Autodesk Inventor part; units mm, degrees
ref_plane "YZ Plane" through (0, 0, 0) normal (1, 0, 0) x (0, 1, 0)
ref_plane "XZ Plane" through (0, 0, 0) normal (0, 1, 0) x (-1, 0, 0)
ref_plane "XY Plane" through (0, 0, 0) normal (0, 0, 1) x (1, 0, 0)
sketch "Sketch1" plane through (0, 0, 0) normal (0, 0, 1) x (1, 0, 0)
  line L0 (0, 0) -> (68.58, 0)
  line L1 (68.58, 0) -> (68.58, 107.95)
  line L2 (68.58, 107.95) -> (0, 107.95)
  line L3 (0, 107.95) -> (0, 0)
  dimension "d0" = 68.58
  dimension "d1" = 107.95
extrude "Extrusion1" add sketch "Sketch1" along normal blind 10
sketch "Sketch2" plane through (0, 0, 10) normal (0, 0, 1) x (1, 0, 0)
  circle A0 centre (34.29, 35.56) radius 30.48
  line L0 (0, 0) -> (68.58, 0)
  line L1 (68.58, 107.95) -> (0, 107.95)
  line L2 (25.1206, 107.95) -> (43.4594, 107.95)
  line L3 (43.4594, 107.95) -> (43.4594, 64.6281)
  line L4 (43.4594, 64.6281) -> (25.1206, 64.6281)
  line L5 (25.1206, 64.6281) -> (25.1206, 107.95)
  circle A1 centre (60.6865, 20.32) radius 5
  circle A2 centre (7.8935, 20.32) radius 5
  line L6 (7.8935, 20.32) -> (34.29, 66.04) construction
  line L7 (34.29, 66.04) -> (60.6865, 20.32) construction
  line L8 (60.6865, 20.32) -> (7.8935, 20.32) construction
  point P0 (34.29, 0)
  point P1 (34.29, 107.95)
  point P2 (57.8397, 16.2095)
  point P3 (62.8229, 24.8406)
  point P4 (10.7403, 16.2095)
  point P5 (5.7571, 24.8406)
  dimension "d4" = 18.3388
  dimension "d5" = 60.96
  dimension "d6" = 35.56
  dimension "d9" = 10
extrude "Extrusion2" cut sketch "Sketch2" against normal blind 7
sketch "Sketch4" plane through (0, 0, 3) normal (0, 0, 1) x (1, 0, 0)
  arc A0 (25.1206, 64.6281) -> (5.7571, 24.8406) centre (34.29, 35.56) ccw
  arc A1 (5.7571, 24.8406) -> (10.7403, 16.2095) centre (7.8935, 20.32) ccw
  arc A2 (10.7403, 16.2095) -> (57.8397, 16.2095) centre (34.29, 35.56) ccw
  arc A3 (57.8397, 16.2095) -> (62.8229, 24.8406) centre (60.6865, 20.32) ccw
  arc A4 (62.8229, 24.8406) -> (43.4594, 64.6281) centre (34.29, 35.56) ccw
  line L0 (43.4594, 107.95) -> (43.4594, 64.6281)
  line L1 (25.1206, 107.95) -> (43.4594, 107.95)
  line L2 (25.1206, 64.6281) -> (25.1206, 107.95)
  line L3 (25.1206, 64.6281) -> (25.1206, 107.95)
  line L4 (43.4594, 107.95) -> (43.4594, 64.6281)
  line L5 (25.1206, 107.95) -> (43.4594, 107.95)
  line L6 (43.4594, 107.95) -> (43.4594, 69.85)
  line L7 (43.4594, 69.85) -> (25.1206, 69.85)
  line L8 (25.1206, 69.85) -> (25.1206, 107.95)
  line L9 (25.1206, 107.95) -> (43.4594, 107.95)
  line L10 (28.1206, 107.95) -> (40.4594, 107.95)
  line L11 (40.4594, 107.95) -> (40.4594, 69.85)
  line L12 (40.4594, 69.85) -> (28.1206, 69.85)
  line L13 (28.1206, 69.85) -> (28.1206, 107.95)
  point P0 (0, 0)
  dimension "d17" = 3
  dimension "d18" = 3
  dimension "d19" = 38.1
extrude "Extrusion4" add sketch "Sketch4" along normal blind 3 contours L13 L1 L11 L7
sketch "Sketch3" plane through (0, 0, 3) normal (0, 0, 1) x (1, 0, 0)
  arc A0 (25.1206, 64.6281) -> (5.7571, 24.8406) centre (34.29, 35.56) ccw
  arc A1 (5.7571, 24.8406) -> (10.7403, 16.2095) centre (7.8935, 20.32) ccw
  arc A2 (10.7403, 16.2095) -> (57.8397, 16.2095) centre (34.29, 35.56) ccw
  arc A3 (57.8397, 16.2095) -> (62.8229, 24.8406) centre (60.6865, 20.32) ccw
  arc A4 (62.8229, 24.8406) -> (43.4594, 64.6281) centre (34.29, 35.56) ccw
  line L0 (43.4594, 107.95) -> (43.4594, 64.6281)
  line L1 (25.1206, 107.95) -> (28.1206, 107.95)
  line L2 (25.1206, 64.6281) -> (25.1206, 107.95)
  line L3 (25.1206, 64.6281) -> (25.1206, 107.95)
  line L4 (25.1206, 107.95) -> (43.4594, 107.95)
  line L5 (43.4594, 107.95) -> (43.4594, 106.95)
  line L6 (43.4594, 106.95) -> (25.1206, 106.95)
  line L7 (25.1206, 106.95) -> (25.1206, 107.95)
  line L8 (40.4594, 107.95) -> (40.4594, 69.85)
  line L9 (40.4594, 69.85) -> (28.1206, 69.85)
  line L10 (28.1206, 69.85) -> (28.1206, 107.95)
  line L11 (40.4594, 107.95) -> (43.4594, 107.95)
  point P0 (0, 0)
  point P1 (40.4594, 106.95)
  point P2 (28.1206, 106.95)
  dimension "d10" = 1
extrude "Extrusion3" add sketch "Sketch3" along normal blind 4.5 contours L2 L1 L10 L6 | L10 L4 L8 L6 | L8 L4 L0 L6
fillet "Fillet1" radius 5 4 edges at (0, 107.95, 5) (68.58, 107.95, 5) (68.58, 0, 5) (0, 0, 5)
chamfer "Chamfer1" distance 2 angle 45 8 edges at (34.29, 107.95, 0) (1.4645, 106.4855, 0) (0, 53.975, 0) (1.4645, 1.4645, 0) (34.29, 0, 0) (67.1155, 1.4645, 0) (68.58, 53.975, 0) (67.1155, 106.4855, 0)
sketch "Sketch6" plane through (0, 0, 10) normal (0, 0, 1) x (1, 0, 0)
  arc A0 (0, 5) -> (5, 0) centre (5, 5) ccw
  line L0 (5, 0) -> (63.58, 0)
  arc A1 (63.58, 0) -> (68.58, 5) centre (63.58, 5) ccw
  line L1 (68.58, 5) -> (68.58, 102.95)
  arc A2 (68.58, 102.95) -> (63.58, 107.95) centre (63.58, 102.95) ccw
  line L2 (63.58, 107.95) -> (43.4594, 107.95)
  line L3 (43.4594, 107.95) -> (43.4594, 64.6281)
  arc A3 (62.8229, 24.8406) -> (43.4594, 64.6281) centre (34.29, 35.56) ccw
  arc A4 (57.8397, 16.2095) -> (62.8229, 24.8406) centre (60.6865, 20.32) ccw
  arc A5 (10.7403, 16.2095) -> (57.8397, 16.2095) centre (34.29, 35.56) ccw
  arc A6 (5.7571, 24.8406) -> (10.7403, 16.2095) centre (7.8935, 20.32) ccw
  arc A7 (25.1206, 64.6281) -> (5.7571, 24.8406) centre (34.29, 35.56) ccw
  line L4 (25.1206, 64.6281) -> (25.1206, 107.95)
  line L5 (25.1206, 107.95) -> (5, 107.95)
  arc A8 (5, 107.95) -> (0, 102.95) centre (5, 102.95) ccw
  line L6 (0, 102.95) -> (0, 5)
  point P0 (0, 0)
hole "Hole2" at (5, 102.95, 10) at (5, 5, 10) at (63.58, 5, 10) at (63.58, 102.95, 10) direction (0, 0, -1) diameter 4 depth 6
sketch "Sketch7" plane through (25.1206, 107.95, 7.5) normal (0, 1, 0) x (1, 0, 0)
  line L0 (3.6694, -5.25) -> (14.6694, -5.25)
  line L1 (14.6694, -5.25) -> (14.6694, 2.75)
  line L2 (14.6694, 2.75) -> (3.6694, 2.75)
  line L3 (3.6694, 2.75) -> (3.6694, -5.25)
  line L4 (-20.1206, 5.5) -> (38.4594, 5.5)
  line L5 (-20.1206, -2.5) -> (-20.1206, 5.5)
  line L6 (0, -2.5) -> (-20.1206, -2.5)
  line L7 (0, -2.5) -> (0, 0)
  line L8 (18.3388, 0) -> (0, 0)
  line L9 (18.3388, 0) -> (18.3388, -2.5)
  line L10 (38.4594, -2.5) -> (18.3388, -2.5)
  line L11 (38.4594, 5.5) -> (38.4594, -2.5)
  line L12 (38.4594, 5.5) -> (-20.1206, 5.5)
  line L13 (3.6694, 2.75) -> (14.6694, 2.75)
  line L14 (14.6694, 2.75) -> (14.6694, 5.5)
  line L15 (14.6694, 5.5) -> (3.6694, 5.5)
  line L16 (3.6694, 5.5) -> (3.6694, 2.75)
  line L17 (3.6694, 5.5) -> (14.6694, 5.5)
  line L18 (14.6694, 5.5) -> (14.6694, 7.5)
  line L19 (14.6694, 7.5) -> (3.6694, 7.5)
  line L20 (3.6694, 7.5) -> (3.6694, 5.5)
  line L21 (38.4594, 7.5) -> (-20.1206, 7.5)
  point P0 (-25.1206, 7.5)
  point P1 (3.6694, -1.25)
  point P2 (0, -1.25)
  point P3 (9.1694, 2.75)
  point P4 (9.1694, 0)
  point P5 (14.6694, 2.75)
  dimension "d36" = 8
  dimension "d37" = 11
extrude "Extrusion5" add sketch "Sketch7" along normal blind 15 and the other way blind 5 contours L16 L4 L14 L2 | L20 L19 L18 L4
sketch "Sketch8" plane through (0, 0, 0) normal (0, 0, -1) x (-1, 0, 0)
  line L0 (-28.79, 107.95) -> (-28.79, 122.95)
  line L1 (-39.79, 105.95) -> (-39.79, 122.95)
  line L2 (-28.79, 119.95) -> (-39.79, 119.95)
  line L3 (-39.79, 119.95) -> (-39.79, 116.95)
  line L4 (-39.79, 116.95) -> (-28.79, 116.95)
  line L5 (-28.79, 116.95) -> (-28.79, 119.95)
  line L6 (-28.79, 111.95) -> (-39.79, 111.95)
  line L7 (-39.79, 111.95) -> (-39.79, 108.95)
  line L8 (-39.79, 108.95) -> (-28.79, 108.95)
  line L9 (-28.79, 108.95) -> (-28.79, 111.95)
  line L10 (-5, 107.95) -> (-28.79, 107.95)
  line L11 (-39.79, 122.95) -> (-28.79, 122.95)
  point P0 (0, 0)
  dimension "d42" = 3
  dimension "d43" = 3
  dimension "d44" = 1
  dimension "d45" = 3
extrude "Extrusion6" cut sketch "Sketch8" against normal blind 1 contours L8 L1 L6 L0 | L4 L1 L2 L0
fillet "Fillet2" radius 2 2 edges at (28.79, 122.95, 2.375) (39.79, 122.95, 2.375)
properties part number "Case Back"
Can you work these out from the model? Positions are in its coordinate system, mm. A direction names the side the tool comes from. Coordinates: 2 decimals unless noted, no trailing zeros. Write each loop counter-clockwise with the first axis right and the second up, starting at its lowest first coordinate (ties: lowest second). Pieces come first, ordered by that corner, then holes.
Q1. Which directions (+Z, -Z, +X, -X, +Y, -Y) give clear straight access to the entire face, cutting with the end or side of a thin tool? Please do faces 4 (the face through (66.23, 2.29, 0.79)), 5 (the face through (64.958, 17.72, 6.549)), 6 (the face through (34, 118, 1)), 7 (the face through (34, 115, 4.75)).
Results found:
face 4: -Z, +X, -Y
face 5: +Z
face 6: -Z, +X, -X
face 7: +Z, +X, -X, +Y
Q2. Imagine slicing it at C-C, the plane y = 47. List the corners of the cut face in (x, z) for me, plus the area to 3 significant figures.
Results found:
outline: (0, 2) - (2, 0) - (66.58, 0) - (68.58, 2) - (68.58, 10) - (62.54, 10) - (62.54, 3) - (6.04, 3) - (6.04, 10) - (0, 10) - close
area: 286 mm2
Q3. Please list where these lines run through material, in increasing order: L1, parallel to X at y = 5, z = 7.65; L2, parallel to X at y = 102.95, z = 6.45; L3, parallel to X at y = 94.5, z = 9.
Results found:
L1: x = 0 to 3, 7 to 61.58, 65.58 to 68.58
L2: x = 0 to 3, 7 to 25.12, 43.46 to 61.58, 65.58 to 68.58
L3: x = 0 to 25.12, 43.46 to 68.58
Q4. Imagine slicing it at A-A, the plane y = 91. List the corners of the cut face in (x, z) for me, plus the area to 3 significant figures.
Results found:
outline: (0, 2) - (2, 0) - (66.58, 0) - (68.58, 2) - (68.58, 10) - (43.46, 10) - (43.46, 3) - (40.46, 3) - (40.46, 6) - (28.12, 6) - (28.12, 3) - (25.12, 3) - (25.12, 10) - (0, 10) - close
area: 590 mm2
Q5. For P1, Ø1.1, axis at x = 38.5, y = 107.5, coming from the +Z side; P2, Ø0.5, axis at x = 34.5, z = 0.5, coming from the -Y side; P3, Ø5, axis at y = 116, z = 1.5, coming from the +X side, each with a flat end and sliding along its axis, tell me the tip position at first contact or that it passes through.
Results found:
P1: stops at z = 7.5
P2: stops at y = 1.25
P3: stops at x = 39.79
Q6. Imagine slicing it at B-B, the plane x = 52.5. List the corners of the cut face in (y, z) for me.
Results found:
outline: (0, 2) - (2, 0) - (105.95, 0) - (107.95, 2) - (107.95, 10) - (60, 10) - (60, 3) - (11.12, 3) - (11.12, 10) - (0, 10) - close
Q7. If we mould it in two halves opening along X, with no side actions, what happens to faces 1 (the face through (34, 121, 0)), 2 (the face through (39.79, 113, 2)), 3 (the face through (25.121, 86, 7))? For each: +X half, -X half, draft (parallel to the pull), parting line (faces both ways), or undercut.
Results found:
face 1: draft
face 2: +X half
face 3: undercut
